Geometry: see drawing. Coordinates: mm, zero at the bounding-box minimum. A direction names the side the tool comes from. Give positions to 0.01 mm unless a question says otherwise; leave off trailing zeros. Order: outer loops, then holes, each group sorted by start corner. A loop starts at its lowest first (then second) coordinate and runs counter-clockwise, first axis right, second up. Notation, with made-up numbers: (-3, 71.25) - (26, 71.25) arc R18 cw to (26, 93.25) - close; hole circle Ø2 at (15.25, 88). An arc over 180 degrees is marked (long way). One line per item, written item: value.
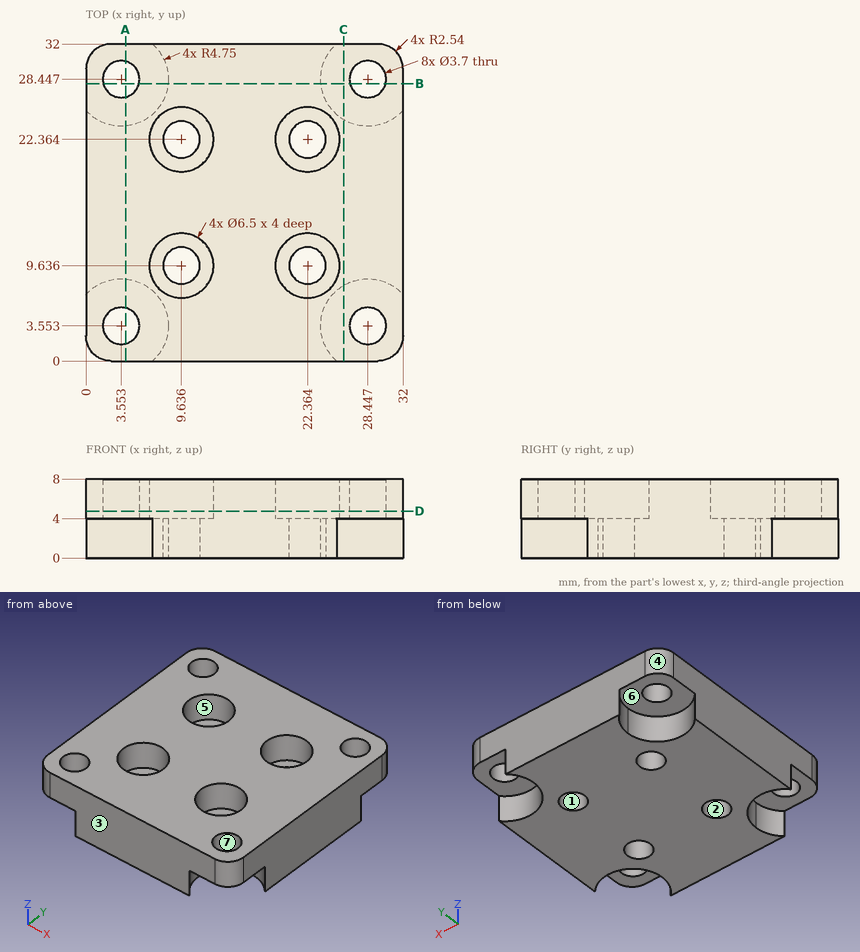
1) Material intervals for line 1 along X through (y, z) = (24.5, 3.5) (1 decimal); line 2 along X through (y, z) = (2, 6); line 3 along Y through (x, z) = (11.5, 6), sorted ascending.
Answers below:
line 1: 0 to 0.9, 6.2 to 25.8, 31.1 to 32
line 2: 0.06 to 2.55, 4.56 to 27.44, 29.45 to 31.94
line 3: 0 to 6.97, 12.3 to 19.7, 25.03 to 32
2) Mould query, pull axis Y, two halves, no side actions, for the marked faces 1, 2, 3 and 4. Classes: released by +Y, released by -Y, zero draft, split by the parting line, or undercut.
Answers below:
face 1: undercut
face 2: undercut
face 3: released by -Y
face 4: released by +Y
3) Set-up query: the marked faces 5, 6 and 7. Return all of +Z, -Z, +X, -X, +Y, -Y with unobstructed straight access to the full face (end or side cutting, diameter ignored); none if empty.
Answers below:
face 5: +Z
face 6: -Z
face 7: +Z, -Z
4) First-contact query: pin 1 (6 mm diameter, centred on x = 9.64, y = 9.64, fed in from +Z); pin 2 (2 mm diameter, centred on x = 22.36, y = 22.36, fed in from -Z); pin 3 (2.5 mm diameter, centred on x = 28, y = 5, fed in from -Z). Flat tips, straight axial feed; report the tip coordinate or a pass-through.
Answers below:
pin 1: z = 4
pin 2: through
pin 3: z = 4
5) Section C-C, the plane x = 26. Return loops of the section in (y, z), then the cut area to 3 significant figures.
Answers below:
outline: (0, 4) - (7.62, 4) - (7.62, 0) - (24.38, 0) - (24.38, 4) - (32, 4) - (32, 8) - (0, 8) - close
area: 195 mm^2
6) Section A-A, the plane x = 4. Return loops of the section in (y, z).
Answers below:
outline: (0, 4) - (1.76, 4) - (1.76, 8) - (0, 8) - close; (5.35, 4) - (8.28, 4) - (8.28, 0) - (23.72, 0) - (23.72, 4) - (26.65, 4) - (26.65, 8) - (5.35, 8) - close; (30.24, 4) - (32, 4) - (32, 8) - (30.24, 8) - close
7) Section D-D, the plane z = 4.75. Count the separate pieces of the cut face and the enclosed holes in it, then the cut area to 3 significant figures.
Answers below:
separate pieces: 1
enclosed holes: 8
area: 843 mm^2
